from build123d import *

# Parameters (mm, degrees)
BOSS_EXTRUDE1_DEPTH     = 5
SKETCH2_W               = 7.5
SKETCH2_H               = 65
BOSS_EXTRUDE2_DEPTH     = 65
FILLET2_R               = 3
SKETCH4_R               = 2.8
SKETCH4_R_2             = 3.5
CUT_EXTRUDE2_DEPTH      = 97.241882775
SKETCH6_R               = 2
CUT_EXTRUDE3_DEPTH      = 80.60841664
SKETCH7_R               = 19.5
CUT_EXTRUDE4_DEPTH      = 3
SKETCH8_W               = 2
SKETCH8_H               = 32.5
BOSS_EXTRUDE3_DEPTH     = 32.5
CUT_EXTRUDE5_DEPTH      = 101.902180353
FILLET3_R               = 3
FILLET4_R               = 1.5
CUT_EXTRUDE6_DEPTH      = 5
FILLET5_R               = 5
CUT_EXTRUDE7_DEPTH      = 101.902180353
CUT_EXTRUDE7_DEPTH_BACK = 101.902180353


with BuildPart() as part:
    # Sketch1 → Boss-Extrude1 (new body)
    with BuildSketch(Plane(origin=(0, 0, 0), x_dir=(1, 0, 0), z_dir=(0, 1, 0))):
        with BuildLine():
            Line((-32.5, 32.5), (27.5, 32.5))
            ThreePointArc((27.5, 32.5), (31.035533906, 31.035533906), (32.5, 27.5))
            Line((32.5, 27.5), (32.5, -27.5))
            ThreePointArc((32.5, -27.5), (31.035533906, -31.035533906), (27.5, -32.5))
            Line((27.5, -32.5), (-32.5, -32.5))
            Line((-32.5, -32.5), (-32.5, 32.5))
        make_face()
    extrude(amount=BOSS_EXTRUDE1_DEPTH)

    # Sketch2 → Boss-Extrude2 (add)
    with BuildSketch(Plane(origin=(0, 5, 0), x_dir=(1, 0, 0), z_dir=(0, 1, 0))):
        with Locations((-28.75, 0)):
            Rectangle(SKETCH2_W, SKETCH2_H)
    extrude(amount=BOSS_EXTRUDE2_DEPTH)

    # Fillet2
    fillet2_edges = [part.edges().sort_by_distance(p)[0] for p in [
        (-32.5, 0, 0),
    ]]
    fillet(fillet2_edges, radius=FILLET2_R)

    # Sketch4 → Cut-Extrude2 (cut, through all)
    with BuildSketch(Plane(origin=(-25, 0, 0), x_dir=(0, 0, -1), z_dir=(1, 0, 0))):
        with Locations((23.57, 61.07)):
            Circle(SKETCH4_R)
        with Locations((-23.57, 61.07)):
            Circle(SKETCH4_R)
        with Locations((-23.57, 13.93)):
            Circle(SKETCH4_R)
        with Locations((23.57, 13.93)):
            Circle(SKETCH4_R)
        with Locations((0, 37.5)):
            Circle(SKETCH4_R_2)
    extrude(amount=-CUT_EXTRUDE2_DEPTH, mode=Mode.SUBTRACT)

    # Sketch6 → Cut-Extrude3 (cut, through all)
    with BuildSketch(Plane(origin=(0, 5, 0), x_dir=(1, 0, 0), z_dir=(0, 1, 0))):
        with Locations(Location((4.5, -10, 0), (0, 0, 270))):
            Circle(SKETCH6_R)
        with Locations(Location((-11.5, -10, 0), (0, 0, 270))):
            Circle(SKETCH6_R)
        with Locations(Location((4.5, 10, 0), (0, 0, 90))):
            Circle(SKETCH6_R)
        with Locations(Location((-11.5, 10, 0), (0, 0, 90))):
            Circle(SKETCH6_R)
    extrude(amount=-CUT_EXTRUDE3_DEPTH, mode=Mode.SUBTRACT)

    # Sketch7 → Cut-Extrude4 (cut)
    with BuildSketch(Plane(origin=(-25, 0, 0), x_dir=(0, 0, -1), z_dir=(1, 0, 0))):
        with Locations((0, 37.5)):
            Circle(SKETCH7_R)
    extrude(amount=-CUT_EXTRUDE4_DEPTH, mode=Mode.SUBTRACT)

    # Sketch8 → Boss-Extrude3 (add)
    with BuildSketch(Plane(origin=(-25, 0, 0), x_dir=(0, 0, -1), z_dir=(1, 0, 0))):
        with Locations((-31.5, 21.25)):
            Rectangle(SKETCH8_W, SKETCH8_H)
        with Locations((31.5, 21.25)):
            Rectangle(SKETCH8_W, SKETCH8_H)
    extrude(amount=BOSS_EXTRUDE3_DEPTH)

    # Sketch9 → Cut-Extrude5 (cut, through all)
    with BuildSketch(Plane.XY.offset(32.5)):
        Polygon((-25, 37.5), (7.5, 5), (7.5, 37.5), align=None)
    extrude(amount=-CUT_EXTRUDE5_DEPTH, mode=Mode.SUBTRACT)

    # Fillet3
    fillet3_edges = [part.edges().sort_by_distance(p)[0] for p in [
        (-25, 5, 0),
    ]]
    fillet(fillet3_edges, radius=FILLET3_R)

    # Fillet4
    fillet4_edges = [part.edges().sort_by_distance(p)[0] for p in [
        (-25, 37.5, -31.5),
        (-25, 22.75, -30.5),
        (-7.25, 5, -30.5),
        (7.5, 5, -31.5),
        (-25, 22.75, 30.5),
        (-24.121320344, 5.878679656, 30.5),
        (-24.121320344, 5.878679656, -30.5),
        (-7.25, 5, 30.5),
        (-25, 37.5, 31.5),
        (7.5, 5, 31.5),
    ]]
    fillet(fillet4_edges, radius=FILLET4_R)

    # Sketch10 → Cut-Extrude6 (cut)
    with BuildSketch(Plane.XZ):
        with BuildLine():
            Line((32.5, -17.85), (-10.5, -17.85))
            Line((-10.5, -17.85), (-10.5, -32.5))
            Line((-10.5, -32.5), (27.5, -32.5))
            ThreePointArc((27.5, -32.5), (31.035533906, -31.035533906), (32.5, -27.5))
            Line((32.5, -27.5), (32.5, -17.85))
        make_face()
        with BuildLine():
            Line((-10.5, 17.85), (32.5, 17.85))
            Line((32.5, 17.85), (32.5, 27.5))
            ThreePointArc((32.5, 27.5), (31.035533906, 31.035533906), (27.5, 32.5))
            Line((27.5, 32.5), (-10.5, 32.5))
            Line((-10.5, 32.5), (-10.5, 17.85))
        make_face()
    extrude(amount=-CUT_EXTRUDE6_DEPTH, mode=Mode.SUBTRACT)

    # Fillet5
    fillet5_edges = [part.edges().sort_by_distance(p)[0] for p in [
        (-10.5, 2.5, -17.85),
        (32.5, 2.5, -17.85),
        (-10.5, 2.5, 17.85),
        (32.5, 2.5, 17.85),
    ]]
    fillet(fillet5_edges, radius=FILLET5_R)

    # Sketch12 → Cut-Extrude7 (cut, two sides: drawn at the far end of the back side and taken through both)
    with BuildSketch(Plane(origin=(0, 0, -32.5), x_dir=(-1, 0, 0), z_dir=(0, 0, -1)).offset(-CUT_EXTRUDE7_DEPTH_BACK)):
        with BuildLine():
            Line((-8.121320344, 5), (10.5, 5))
            Line((10.5, 5), (24.857345269, 37.482873932))
            ThreePointArc((24.857345269, 37.482873932), (24.727295275, 37.258913069), (24.560660172, 37.060660172))
            Line((24.560660172, 37.060660172), (-7.060660172, 5.439339828))
            ThreePointArc((-7.060660172, 5.439339828), (-7.547295195, 5.114180701), (-8.121320344, 5))
        make_face()
    extrude(amount=CUT_EXTRUDE7_DEPTH + CUT_EXTRUDE7_DEPTH_BACK, mode=Mode.SUBTRACT)


solid = part.part
The listing builds one solid part. Answer for the finished solid, in the listing's coordinates (mm). A direction names the side the tool comes from. Coordinates: 2 decimals unless noted, no trailing zeros. Loops run counter-clockwise (first coordinate to the right, second up) from the corner with the lowest first, then second, coordinate; pieces in that order, holes last. Notation, with made-up numbers: M -13,86 L -7,86 A20 cw -7,105 Z; hole C 4,41.25 d2. An arc over 180 degrees is marked long. Answer in a Markdown table with one row per item.
1) Given pin 1 (6.5 mm diameter, centred on y = 61.07, z = -23.57, fed in from +X); pin 2 (16.5 mm diameter, centred on x = 15.5, z = 0, fed in from +Y); pin 3 (1.5 mm diameter, centred on x = 11, y = 2, fed in from +Z), each flat-ended and moving along its own axis, determine where each tip first touches the part or whether it passes through.
Answers below:
| item | result |
|---|---|
| pin 1 | x = -25 |
| pin 2 | y = 5 |
| pin 3 | z = 17.85 |
2) Which of the six approach directions +Z, -Z, +X, -X, +Y, -Y give full straight-line access (tool end or side, diameter ignored) to faces 1 (the flat face through (11, 2, 17.85)), 2 (the flat face through (-25, 52, -14)), 3 (the flat face through (11, 2, -17.85))?
Answers below:
| item | result |
|---|---|
| face 1 | +Z, +X, +Y, -Y |
| face 2 | +X, +Y |
| face 3 | -Z, +X, +Y, -Y |
3) Find section D-D (z = -10). Determine the outline of the cut face in (x, y).
Answers below:
| item | result |
|---|---|
| outline | M -32.5,3 A3 ccw -29.5,0 L -13.5,0 L -13.5,5 L -22,5 A3 cw -25,8 L -25,20.76 L -28,20.76 L -28,54.24 L -25,54.24 L -25,70 L -32.5,70 Z; M -9.5,0 L 2.5,0 L 2.5,5 L -9.5,5 Z; M 6.5,0 L 32.5,0 L 32.5,5 L 6.5,5 Z |
4) Find section A-A (y = 61.07). Determine the outline of the cut face in (x, z), then the cut area to 4 significant figures.
Answers below:
| item | result |
|---|---|
| outline | M -32.5,-32.5 L -25,-32.5 L -25,-26.37 L -32.5,-26.37 Z; M -32.5,-20.77 L -25,-20.77 L -25,20.77 L -32.5,20.77 Z; M -32.5,26.37 L -25,26.37 L -25,32.5 L -32.5,32.5 Z |
| area | 403.5 mm^2 |
5) Determine the mould class of faces 4 (the cylindrical face through (-26.479, 18.464, 4.227)), 5 (the cylindrical face through (-30, 41, 0)), 6 (the flat face through (-10.5, 2, -28)), 7 (the flat face through (-5, 0, 0)) for opening direction Y: released by +Y, released by -Y, zero draft, split by the parting line, or undercut.
Answers below:
| item | result |
|---|---|
| face 4 | undercut |
| face 5 | undercut |
| face 6 | zero draft |
| face 7 | released by -Y |
6) Find section C-C (y = 36). Determine the outline of the cut face in (x, z), then the cut area to 3 significant figures.
Answers below:
| item | result |
|---|---|
| outline | M -32.5,-32.5 L -24.2,-32.5 L -24.2,-30.33 A1.5 cw -25,-29 L -25,-19.44 L -28,-19.44 L -28,-3.16 L -32.5,-3.16 Z; M -32.5,3.16 L -28,3.16 L -28,19.44 L -25,19.44 L -25,29 A1.5 cw -24.2,30.33 L -24.2,32.5 L -32.5,32.5 Z |
| area | 346 mm^2 |
7) Find section B-B (z = 28). Determine the outline of the cut face in (x, y), then the cut area to 4 significant figures.
Answers below:
| item | result |
|---|---|
| outline | M -32.5,3 A3 ccw -29.5,0 L -10.5,0 L -10.5,5 L -22,5 A3 cw -25,8 L -25,70 L -32.5,70 Z |
| area | 597.5 mm^2 |
8) Find the intervals of material crossed by probe 1 along Y at (x, z) = (-29.5, 23.57); probe 2 along X at (y, z) = (3.2, 10); probe 3 along Y at (x, z) = (1, 14.5), in increasing order.
Answers below:
| item | result |
|---|---|
| probe 1 | 0 to 11.13, 16.73 to 58.27, 63.87 to 70 |
| probe 2 | -32.5 to -13.5, -9.5 to 2.5, 6.5 to 32.5 |
| probe 3 | 0 to 5 |
